For this review, take the finished solid that the model builds, in its own axes (mm). Face numbers are marked on the shaded views. A direction names the side the tool comes from. Coordinates: 2 decimals unless noted, no trailing zeros. Loops run counter-clockwise (first coordinate to the right, second up) from the corner with the lowest first, then second, coordinate; pieces in that order, holes last. Notation, with made-up numbers: M 19.25,-1 L 57.25,-1 A20 cw 57.25,14 Z; hole C -32,59.25 d5. An arc over 180 degrees is marked long. Put each result on its own line as item: value.
```python
from build123d import *

# Parameters (mm, degrees)
BOSS_EXTRUDE1_DEPTH = 3.85
CHAMFER1_SIZE       = 1


with BuildPart() as part:
    # Sketch1 → Boss-Extrude1 (new body)
    with BuildSketch(Plane(origin=(0, 0, 0), x_dir=(1, 0, 0), z_dir=(0, 1, 0))):
        with BuildLine():
            Line((-17.644097819, 33.396892859), (-14.745475234, 34.423348951))
            Line((-14.745475234, 34.423348951), (-13.076440938, 29.710141496))
            Line((-13.076440938, 29.710141496), (-9.447271197, 30.995297904))
            Line((-9.447271197, 30.995297904), (-11.116305493, 35.708505359))
            Line((-11.116305493, 35.708505359), (-8.217682908, 36.734961451))
            ThreePointArc((-8.217682908, 36.734961451), (-3.473682306, 18.55498598), (-1.876973594, -0.165793148))
            Line((-1.876973594, -0.165793148), (-4.951973594, -0.165793148))
            Line((-4.951973594, -0.165793148), (-4.951973594, 4.834206852))
            Line((-4.951973594, 4.834206852), (-8.801973594, 4.834206852))
            Line((-8.801973594, 4.834206852), (-8.801973594, -0.165793148))
            Line((-8.801973594, -0.165793148), (-11.876973594, -0.165793148))
            ThreePointArc((-11.876973594, -0.165793148), (-13.329242897, 16.861490941), (-17.644097819, 33.396892859))
        make_face()
    extrude(amount=BOSS_EXTRUDE1_DEPTH)

    # Chamfer1
    chamfer1_edges = [part.edges().sort_by_distance(p)[0] for p in [
        (-14.745475234, 1.925, -34.423348951),
        (-11.116305493, 1.925, -35.708505359),
        (-4.951973594, 1.925, 0.165793148),
        (-8.801973594, 1.925, 0.165793148),
    ]]
    chamfer(chamfer1_edges, length=CHAMFER1_SIZE)


solid = part.part
```
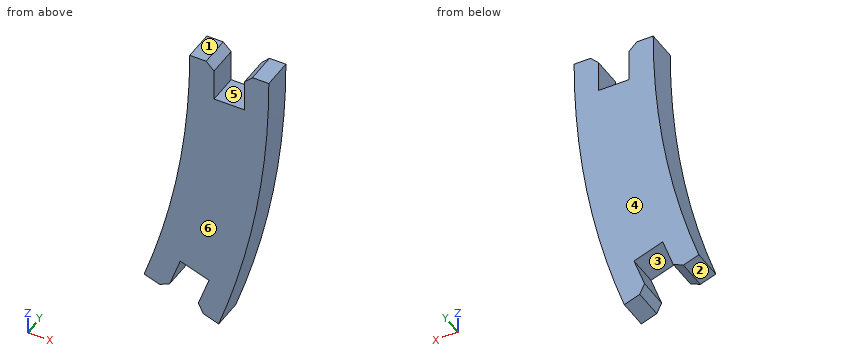
(1) Add section C-C (x = -3). Write out the cut boundary in (y, z), plus the area to 3 significant figures.
Determined:
outline: M 0,-15.55 L 3.85,-15.55 L 3.85,0.17 L 0,0.17 Z
area: 60.5 mm^2
(2) Wall thickness on line 1 along X through (y, z) = (1.45, -1); line 2 along X through (y, z) = (1.7, -31.5); line 3 along Z through (x, y) = (-8.5, 2): over which ranges is each line inside the solid? List them lowest first. Write a range as [from, to].
Determined:
line 1: x = [-11.88, -8.8], [-4.95, -1.88]
line 2: x = [-16.99, -13.71], [-9.63, -6.51]
line 3: z = [-36.63, -4.83]
(3) Add section B-B (y = 2.2). Write out the cut boundary in (x, z).
Determined:
outline: M -17.64,-33.4 L -15.69,-34.09 L -14.41,-33.48 L -13.08,-29.71 L -9.45,-31 L -10.78,-34.77 L -10.17,-36.04 L -8.22,-36.73 A110.55 ccw -1.88,0.17 L -3.95,0.17 L -4.95,-0.83 L -4.95,-4.83 L -8.8,-4.83 L -8.8,-0.83 L -9.8,0.17 L -11.88,0.17 A100.55 cw Z
(4) For pin 1 (1.5 mm diameter, centred on y = 3, z = -12, fed in from +X); pin 2 (1.5 mm diameter, centred on y = 3, z = -6, fed in from -X); pin 3 (1 mm diameter, centred on y = 2, z = -8, fed in from +X); pin 4 (1.5 mm diameter, centred on x = -4, y = 3, fed in from +Z), all flat-tipped, find the tip position at first contact; note any pin that passes through.
Determined:
pin 1: stops at x = -2.47
pin 2: stops at x = -12.12
pin 3: stops at x = -2.14
pin 4: stops at z = 0.17
(5) Add section A-A (z = -2.5). Write out the cut boundary in (x, y).
Determined:
outline: M -11.91,0 L -8.8,0 L -8.8,3.85 L -11.91,3.85 Z; M -4.95,0 L -1.91,0 L -1.91,3.85 L -4.95,3.85 Z
(6) Tool access review of the marked faces 5 and 6: name each direction out of +Z, -Z, +X, -X, +Y, -Y from which nothing blocks a thin tool from reaching the whole face with its end or side.
Determined:
face 5: +Z, +Y, -Y
face 6: +Z, -Z, +X, -X, -Y
(7) Add section D-D (z = -33). Write out the cut boundary in (x, y), plus the area to 3 significant figures.
Determined:
outline: M -17.5,0 L -14.24,0 L -14.24,3.85 L -17.5,3.85 Z; M -10.16,0 L -6.97,0 L -6.97,3.85 L -10.16,3.85 Z
area: 24.8 mm^2
(8) Draft analysis for pull direction Z (two halves, no side actions). For the marked faces 1, 2, 3 and 4, state which applies: +Z half, -Z half, draft (parallel to the pull), parting line (faces both ways), or undercut.
Determined:
face 1: +Z half
face 2: -Z half
face 3: undercut
face 4: draft
